Input: part model. Units: mm. Frame: model coordinates. Face numbers are marked on the shaded views. A direction names the side the tool comes from. Round coordinates to 2 decimals unless told otherwise and drop trailing zeros. Order: outer loops, then holes, each group sorted by start corner. A loop starts at its lowest first (then second) coordinate and runs counter-clockwise, first axis right, second up. Notation, with made-up numbers: (9.5, -13) - (41.5, -13) arc R24 ccw to (41.5, -2) - close; hole circle Ø11 at (-29.75, 64). An arc over 180 degrees is marked (long way). One line per item, written item: value. Start each with the question number.
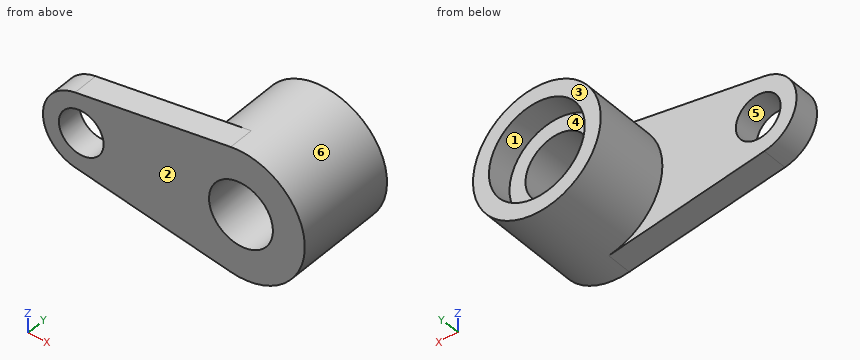
from build123d import *

# Parameters (mm, degrees)
EXTRUDE_3_DEPTH     = 8
SKETCH_5_R          = 20
EXTRUDE_4_DEPTH     = 32
SKETCH_7_R          = 15
CUT_EXTRUDE_1_DEPTH = 8
SKETCH_8_R          = 10
CUT_EXTRUDE_2_DEPTH = 38
SKETCH_9_R          = 7
CUT_EXTRUDE_4_DEPTH = 18


with BuildPart() as part:
    # 草图2 → 凸台-拉伸3 (new body)
    with BuildSketch(Plane(origin=(0, 0, 0), x_dir=(1, 0, 0), z_dir=(0, 1, 0))):
        with BuildLine():
            Line((-3.2, 19.742340287), (-51.92, 11.845404172))
            ThreePointArc((-51.92, 11.845404172), (-62, 0), (-51.92, -11.845404172))
            Line((-51.92, -11.845404172), (-3.2, -19.742340287))
            ThreePointArc((-3.2, -19.742340287), (20, 0), (-3.2, 19.742340287))
        make_face()
    extrude(amount=EXTRUDE_3_DEPTH)

    # 草图5 → 凸台-拉伸4 (add)
    with BuildSketch(Plane(origin=(0, 0, 0), x_dir=(1, 0, 0), z_dir=(0, 1, 0))):
        with Locations(Location((0, 0, 0), (0, 0, 99.206896221))):
            Circle(SKETCH_5_R)
    extrude(amount=EXTRUDE_4_DEPTH)

    # 草图7 → 切除-拉伸1 (cut)
    with BuildSketch(Plane(origin=(0, 32, 0), x_dir=(1, 0, 0), z_dir=(0, 1, 0))):
        with Locations(Location((0, 0, 0), (0, 0, 270))):
            Circle(SKETCH_7_R)
    extrude(amount=-CUT_EXTRUDE_1_DEPTH, mode=Mode.SUBTRACT)

    # 草图8 → 切除-拉伸2 (cut)
    with BuildSketch(Plane(origin=(0, 0, 0), x_dir=(1, 0, 0), z_dir=(0, 1, 0))):
        with Locations(Location((0, 0, 0), (0, 0, 270))):
            Circle(SKETCH_8_R)
    extrude(amount=CUT_EXTRUDE_2_DEPTH, mode=Mode.SUBTRACT)

    # 草图9 → 切除-拉伸4 (cut)
    with BuildSketch(Plane(origin=(0, 0, 0), x_dir=(1, 0, 0), z_dir=(0, 1, 0))):
        with Locations(Location((-50, 0, 0), (0, 0, 270))):
            Circle(SKETCH_9_R)
    extrude(amount=CUT_EXTRUDE_4_DEPTH, mode=Mode.SUBTRACT)


solid = part.part
Item 1: Section query A-A on x = 0. Return loops of the section in (y, z).
Item 2: Section query B-B on z = 0. Return loops of the section in (x, y), and give its area (3 significant figures).
Item 3: Pull-direction query (Z, two-part tool) for the marked faces 3, 4, 5 and 6; classes: released by +Z, released by -Z, zero draft, split by the parting line, or undercut.
Item 4: Line query: L1, parallel to X at y = 5.75, z = 0; L2, parallel to X at y = 5.5, z = 4; L3, parallel to Z at x = 0, y = 8. Output: solid intervals per line, ascending.
Item 5: First-contact query: pin 1 Ø1.5 at (y, z) = (6, -10) entering from -X; pin 2 Ø2 at (x, y) = (-15, 4.5) entering from -Z; pin 3 Ø2 at (x, y) = (4, 23.5) entering from -Z; pin 4 Ø18 at (x, z) = (-50, 0) entering from -Y. Flat tips, straight axial feed; report the tip coordinate or a pass-through.
Item 6: Section query D-D on z = -8. Return loops of the section in (x, y).
Item 7: Section query C-C on y = 6.5. Return loops of the section in (x, z).
Item 8: Reachability of the marked faces 1 and 2 from +Z, -Z, +X, -X, +Y, -Y: full face, straight path, thin tool, end or side. Return the list, or none.
Geometry results:
1. outline: (0, -20) - (32, -20) - (32, -15) - (24, -15) - (24, -10) - (0, -10) - close; (0, 10) - (24, 10) - (24, 15) - (32, 15) - (32, 20) - (0, 20) - close
2. outline: (-62, 0) - (-57, 0) - (-57, 8) - (-62, 8) - close; (-43, 0) - (-10, 0) - (-10, 24) - (-15, 24) - (-15, 32) - (-20, 32) - (-20, 8) - (-43, 8) - close; (10, 0) - (20, 0) - (20, 32) - (15, 32) - (15, 24) - (10, 24) - close
2. area: 784 mm^2
3. face 3: zero draft
3. face 4: undercut
3. face 5: undercut
3. face 6: split by the parting line
4. L1: x = -62 to -57, -43 to -10, 10 to 20
4. L2: x = -61.31 to -55.74, -44.26 to -9.17, 9.17 to 19.6
4. L3: z = -20 to -10, 10 to 20
5. pin 1: stops at x = -57.64
5. pin 2: stops at z = -17.99
5. pin 3: stops at z = -19.77
5. pin 4: stops at y = 0
6. outline: (-58.94, 0) - (-6, 0) - (-6, 24) - (-12.69, 24) - (-12.69, 32) - (-18.33, 32) - (-18.33, 8) - (-58.94, 8) - close; (6, 0) - (18.33, 0) - (18.33, 32) - (12.69, 32) - (12.69, 24) - (6, 24) - close
7. outline: (-51.92, -11.85) - (-3.2, -19.74) arc R20 ccw (long way) to (-3.2, 19.74) - (-51.92, 11.85) arc R12 ccw to start; hole circle Ø14 at (-50, 0); hole circle Ø20 at (0, 0)
8. face 1: +Y
8. face 2: +Z, -Z, +X, -X, -Y
